For this review, take the finished solid that the model builds, in its own axes (mm). Face numbers are marked on the shaded views. A direction names the side the tool comes from. Coordinates: 2 decimals unless noted, no trailing zeros. Order: outer loops, then holes, each group sorted by start corner. A loop starts at its lowest first (then second) coordinate and runs counter-clockwise, first axis right, second up. Notation, with made-up numbers: (21, -12.5) -> (53, -12.5) arc R20 ccw to (53, 7.5) -> close; hole circle Ø9 at (72.5, -5.5). An arc over 180 degrees is marked (long way). Write item = value, one per line. Start each with the question number.
1) Draft analysis for pull direction X (two halves, no side actions). For the marked faces 1, 2, 3 and 4, state which applies: +X half, -X half, draft (parallel to the pull), parting line (faces both ways), or undercut.
2) Consider section B-B on z = -10. Give the boundary of the cut face in (x, y).
3) Consider section D-D on y = -2.25. Give the boundary of the cut face in (x, z), and give its area (3 significant figures).
4) Consider section A-A on y = 0.4. Give the boundary of the cut face in (x, z).
5) Machinability: for the marked faces 5 and 6, which of the approach directions +Z, -Z, +X, -X, +Y, -Y give a long, thin tool a straight path to every point of the face, cutting with its end or side? Answer none if there is none.
6) Consider section C-C on x = -5.5. Give the boundary of the cut face in (y, z).
7) Insertion check: pin 1 Ø1.5 at (x, z) = (6.5, -2) entering from +Y. The pin has a flat end and moves straight along its axis. Give the tip position at first contact, or say it passes through.
8) Wall thickness on probe 1 along X at (y, z) = (1.8, 5.5); probe 2 along Z at (x, y) = (7.75, -0.8); probe 3 along Z at (x, y) = (-4.5, 2.3): over which ranges is each line inside the solid? List them lowest first. Write a range as [from, to].
from build123d import *

# Parameters (mm, degrees)
SALIENTE_EXTRUIR1_DEPTH = 3
SALIENTE_EXTRUIR2_DEPTH = 3
CROQUIS3_W              = 3
CROQUIS3_H              = 6
CORTAR_EXTRUIR3_DEPTH   = 4
CROQUIS4_W              = 2
CROQUIS4_H              = 6
CORTAR_EXTRUIR4_DEPTH   = 4


with BuildPart() as part:
    # Croquis1 → Saliente-Extruir1 (new body)
    with BuildSketch(Plane(origin=(0, 0, 0), x_dir=(1, 0, 0), z_dir=(0, 1, 0))):
        with BuildLine():
            Line((-4, 12.8), (-9.3, 12.8))
            ThreePointArc((-9.3, 12.8), (-10.007106781, 12.507106781), (-10.3, 11.8))
            Line((-10.3, 11.8), (-10.3, -11.8))
            ThreePointArc((-10.3, -11.8), (-10.007106781, -12.507106781), (-9.3, -12.8))
            Line((-9.3, -12.8), (9.3, -12.8))
            ThreePointArc((9.3, -12.8), (10.007106781, -12.507106781), (10.3, -11.8))
            Line((10.3, -11.8), (10.3, 11.8))
            ThreePointArc((10.3, 11.8), (10.007106781, 12.507106781), (9.3, 12.8))
            Line((9.3, 12.8), (4, 12.8))
            Line((4, 12.8), (4, 11.3))
            Line((4, 11.3), (8.8, 11.3))
            Line((8.8, 11.3), (8.8, -11.3))
            Line((8.8, -11.3), (-8.8, -11.3))
            Line((-8.8, -11.3), (-8.8, 11.3))
            Line((-8.8, 11.3), (-4, 11.3))
            Line((-4, 11.3), (-4, 12.8))
        make_face()
    extrude(amount=SALIENTE_EXTRUIR1_DEPTH)

    # Croquis1_3 → Saliente-Extruir2 (add)
    with BuildSketch(Plane(origin=(0, 0, 0), x_dir=(1, 0, 0), z_dir=(0, 1, 0))):
        with BuildLine():
            ThreePointArc((-9.3, 12.8), (-10.007106781, 12.507106781), (-10.3, 11.8))
            Line((-10.3, 11.8), (-10.3, -11.8))
            ThreePointArc((-10.3, -11.8), (-10.007106781, -12.507106781), (-9.3, -12.8))
            Line((-9.3, -12.8), (9.3, -12.8))
            ThreePointArc((9.3, -12.8), (10.007106781, -12.507106781), (10.3, -11.8))
            Line((10.3, -11.8), (10.3, 11.8))
            ThreePointArc((10.3, 11.8), (10.007106781, 12.507106781), (9.3, 12.8))
            Line((9.3, 12.8), (-9.3, 12.8))
        make_face()
    extrude(amount=-SALIENTE_EXTRUIR2_DEPTH)

    # Croquis3 → Cortar-Extruir3 (cut)
    with BuildSketch(Plane(origin=(10.3, 0, 0), x_dir=(0, 0, -1), z_dir=(1, 0, 0))):
        with Locations((-9.8, 0)):
            Rectangle(CROQUIS3_W, CROQUIS3_H)
    extrude(amount=-CORTAR_EXTRUIR3_DEPTH, mode=Mode.SUBTRACT)

    # Croquis4 → Cortar-Extruir4 (cut)
    with BuildSketch(Plane.XY.offset(12.8)):
        with Locations((-7.8, 0)):
            Rectangle(CROQUIS4_W, CROQUIS4_H)
    extrude(amount=-CORTAR_EXTRUIR4_DEPTH, mode=Mode.SUBTRACT)


solid = part.part
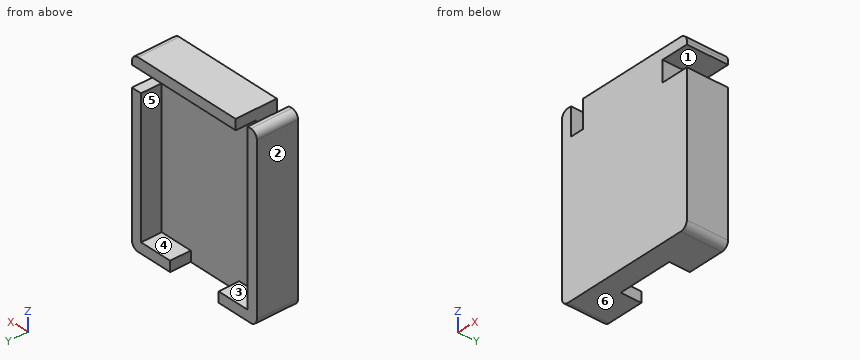
Answer sheet:
q1.face_1 = draft
q1.face_2 = -X half
q1.face_3 = undercut
q1.face_4 = undercut
q2.outline = (-10.3, -3) -> (10.3, -3) -> (10.3, 3) -> (8.8, 3) -> (8.8, 0) -> (-8.8, 0) -> (-8.8, 3) -> (-10.3, 3) -> close
q3.outline = (-10.3, -11.8) arc R1 ccw to (-9.3, -12.8) -> (9.3, -12.8) arc R1 ccw to (10.3, -11.8) -> (10.3, 8.3) -> (6.3, 8.3) -> (6.3, 11.3) -> (10.3, 11.3) -> (10.3, 11.8) arc R1 ccw to (9.3, 12.8) -> (-6.8, 12.8) -> (-6.8, 8.8) -> (-8.8, 8.8) -> (-8.8, 12.8) -> (-9.3, 12.8) arc R1 ccw to (-10.3, 11.8) -> close
q3.area = 507 mm2
q4.outline = (-10.3, -11.8) arc R1 ccw to (-9.3, -12.8) -> (-4, -12.8) -> (-4, -11.3) -> (-8.8, -11.3) -> (-8.8, 12.8) -> (-9.3, 12.8) arc R1 ccw to (-10.3, 11.8) -> close; (-6.8, 11.3) -> (10.3, 11.3) -> (10.3, 11.8) arc R1 ccw to (9.3, 12.8) -> (-6.8, 12.8) -> close; (4, -12.8) -> (9.3, -12.8) arc R1 ccw to (10.3, -11.8) -> (10.3, 8.3) -> (8.8, 8.3) -> (8.8, -11.3) -> (4, -11.3) -> close
q5.face_5 = +Y
q5.face_6 = -Z, +X, -X, +Y, -Y
q6.outline = (-3, -12.8) -> (3, -12.8) -> (3, -11.3) -> (0, -11.3) -> (0, 11.3) -> (3, 11.3) -> (3, 12.8) -> (-3, 12.8) -> close
q7.pin_1 = 0
q8.probe_1 = [-10.3, -8.8], [8.8, 10.3]
q8.probe_2 = [-12.8, 8.3], [11.3, 12.8]
q8.probe_3 = [-12.8, -11.3], [11.3, 12.8]
